Check sheet for the drawn part. Datum: minimum x, y, z corner. Units: mm. Round coordinates to 2 decimals unless told otherwise and drop trailing zeros. Write each loop counter-clockwise with the first axis right and the second up, starting at its lowest first coordinate (ties: lowest second). Pieces come first, ordered by that corner, then holes.
Item 1: Material ranges on line 1 (Z direction, x = 1.5, y = 2.3); line 2 (X direction, y = 1.9, z = 135.5); line 3 (X direction, y = 1.45, z = 112.5), recorded low to high.
Item 2: Cross-section at B-B on z = 20. Enter the section's corners in (x, y).
Item 3: Cross-section at A-A on y = 1.6. Count the separate pieces of the cut face and the enclosed holes in it, plus the area to 3 significant figures.
Item 4: Go/stop test with flat-tipped pins: pin 1 Ø0.9 at (x, y) = (1, 1) entering from +Z; pin 2 Ø0.9 at (y, z) = (2, 118) entering from -X; pin 3 Ø1.5 at (x, y) = (28.5, 1) entering from +Z. Record where each tip stops, or that it passes through.
Item 5: Cross-section at C-C on x = 79.5. Enter the section's corners in (y, z).
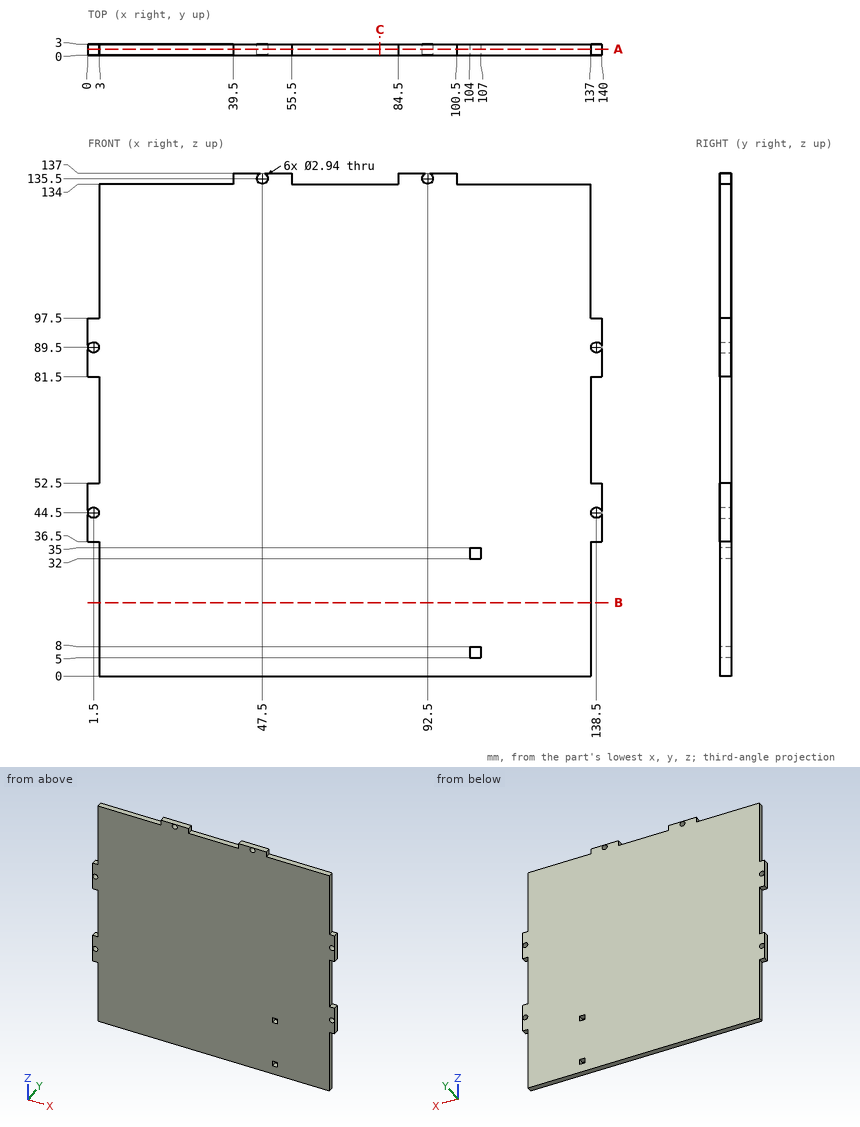
Response values:
1. line 1: z = 36.5 to 43.03, 45.97 to 52.5, 81.5 to 88.03, 90.97 to 97.5
1. line 2: x = 39.5 to 46.03, 48.97 to 55.5, 84.5 to 91.03, 93.97 to 100.5
1. line 3: x = 3 to 137
2. outline: (3, 0) - (137, 0) - (137, 3) - (3, 3) - close
3. separate pieces: 1
3. enclosed holes: 8
3. area: 18,200 mm2
4. pin 1: stops at z = 97.5
4. pin 2: stops at x = 3
4. pin 3: stops at z = 134
5. outline: (0, 0) - (3, 0) - (3, 134) - (0, 134) - close
